Autodesk Inventor part; units mm, degrees
ref_plane "YZ Plane" through (0, 0, 0) normal (1, 0, 0) x (0, 1, 0)
ref_plane "XZ Plane" through (0, 0, 0) normal (0, 1, 0) x (-1, 0, 0)
ref_plane "XY Plane" through (0, 0, 0) normal (0, 0, 1) x (1, 0, 0)
ref_plane "Work Plane1" through (0, 0, 0) normal (0, 0, -1) x (-1, 0, 0)
sketch "Sketch16" plane through (0, 0, 0) normal (0, 0, -1) x (-1, 0, 0)
  line L0 (0, 0) -> (-76.2, 0)
  line L1 (-76.2, 0) -> (-101.6, 0)
  line L2 (-101.6, 0) -> (-101.6, 50.8)
  line L3 (-101.6, 50.8) -> (-76.2, 50.8)
  line L4 (-76.2, 50.8) -> (-76.2, 0)
  line L5 (-78.74, 48.26) -> (-99.06, 48.26)
  line L6 (-99.06, 48.26) -> (-99.06, 2.54)
  line L7 (-99.06, 2.54) -> (-78.74, 2.54)
  line L8 (-78.74, 2.54) -> (-78.74, 48.26)
  dimension "d54" = 25.4
  dimension "d55" = 50.8
  dimension "d56" = 2.54
  dimension "d57" = 2.54
  dimension "d58" = 2.54
  dimension "d59" = 2.54
extrude "Extrusion13" add sketch "Sketch16" against normal blind 152.4
ref_plane "Work Plane4" through (0, 0, 0) normal (0, 0, -1) x (-1, 0, 0)
ref_plane "Work Plane3" through (0, 0, 0) normal (0, -1, 0) x (1, 0, 0)
sketch "Sketch20" plane through (0, 0, 0) normal (0, -1, 0) x (1, 0, 0)
  circle A0 centre (88.9, 12.7) radius 2.5797
  circle A1 centre (63.5, 12.7) radius 2.5797
  circle A2 centre (38.1, 12.7) radius 2.5797
  line L0 (0, 25.4) -> (76.2, 25.4)
  circle A3 centre (88.9, 38.1) radius 2.5797
  circle A4 centre (88.9, 63.5) radius 2.5797
  line L1 (76.2, 25.4) -> (76.2, 152.4)
  line L2 (101.6, 0) -> (101.6, 152.4)
  point P0 (0, 0)
  dimension "d71" = 12.7
  dimension "d72" = 12.7
  dimension "d73" = 12.7
  dimension "d74" = 5.1594
  dimension "d75" = 5.1594
  dimension "d76" = 5.1594
  dimension "d77" = 12.7
  dimension "d78" = 12.7
  dimension "d79" = 5.1594
  dimension "d80" = 5.1594
  dimension "d81" = 12.7
  dimension "d82" = 25.4
  dimension "d83" = 25.4
  dimension "d84" = 25.4
  dimension "d85" = 25.4
extrude "Extrusion16" cut sketch "Sketch20" against normal blind 76.2
ref_plane "Work Plane2" through (0, 50.8, 25.4) normal (0, 1, 0) x (1, 0, 0)
sketch "Sketch24" plane through (0, 50.8, 25.4) normal (0, 1, 0) x (1, 0, 0)
  circle A0 centre (88.9, -114.3) radius 2.5797
  circle A1 centre (88.9, -88.9) radius 2.5797
  line L0 (101.6, -127) -> (76.2, -127)
  line L1 (76.2, 0) -> (76.2, -127)
  point P0 (0, 25.4)
  dimension "d112" = 12.7
  dimension "d113" = 25.4
  dimension "d114" = 5.1594
  dimension "d115" = 5.1594
  dimension "d116" = 12.7
  dimension "d117" = 12.7
extrude "Extrusion20" cut sketch "Sketch24" against normal blind 50.8
sketch "Sketch25" plane through (101.6, 0, 0) normal (1, 0, 0) x (0, 0, -1)
  point P0 (0, 0)
equation "\"d56\" = d48"
equation "\"d57\" = d48"
equation "\"d58\" = d48"
equation "\"d59\" = d48"
equation "\"d72\" = d71"
equation "\"d73\" = d71"
equation "\"d75\" = d74"
equation "\"d76\" = d74"
equation "\"d77\" = d71"
equation "\"d78\" = d71"
equation "\"d79\" = d74"
equation "\"d80\" = d74"
equation "\"d81\" = d71"
equation "\"d83\" = d82"
equation "\"d84\" = d82"
equation "\"d85\" = d82"
equation "\"d115\" = d114"
properties part number "right arm"
Source: CAD feature listing. Evaluate the final solid. Frame: model axes, mm. A direction names the side the tool comes from. Round coordinates to 2 decimals unless told otherwise and drop trailing zeros. Loops run counter-clockwise (first coordinate to the right, second up) from the corner with the lowest first, then second, coordinate; pieces in that order, holes last. Notation, with made-up numbers: (39, 84.5) - (63, 84.5) arc R22 ccw to (63, 106.5) - close; hole circle Ø5 at (34, 36.5). An arc over 180 degrees is marked (long way). Write item = value, one per line. Start each with the question number.
Item 1: Section query C-C on z = 139.7. Output: boundary loops of the cut face in (x, y).
Item 2: Material intervals for line 1 (Z direction, x = 88.9, y = 49.2); line 2 (X direction, y = 19.5, z = 93); line 3 (Y direction, x = 82.25, z = 89), sorted ascending.
Item 3: Mould query, pull axis X, two halves, no side actions, for faces 3 (the face through (101.6, 25, 75)), 4 (the face through (99.3, 27.4, 152.4)), 5 (the face through (89, 48.26, 75)). Classes: released by +X, released by -X, zero draft, split by the parting line, or undercut.
Item 4: Section query D-D on z = 119.5. Output: boundary loops of the cut face in (x, y).
Item 5: Section query B-B on x = 96.5. Output: boundary loops of the cut face in (y, z).
Item 6: Section query A-A on y = 43. Output: boundary loops of the cut face in (x, z).
Item 7: Reachability of faces 1 (the face through (99.06, 26, 75)), 2 (the face through (88.564, 1.252, 66.058)) from +Z, -Z, +X, -X, +Y, -Y: full face, straight path, thin tool, end or side. Return the list, or none.
Results list:
q1.outline = (76.2, 0) - (86.32, 0) - (86.32, 2.54) - (78.74, 2.54) - (78.74, 48.26) - (86.32, 48.26) - (86.32, 50.8) - (76.2, 50.8) - close; (91.48, 0) - (101.6, 0) - (101.6, 50.8) - (91.48, 50.8) - (91.48, 48.26) - (99.06, 48.26) - (99.06, 2.54) - (91.48, 2.54) - close
q2.line_1 = 0 to 10.12, 15.28 to 35.52, 40.68 to 60.92, 66.08 to 111.72, 116.88 to 137.12, 142.28 to 152.4
q2.line_2 = 76.2 to 78.74, 99.06 to 101.6
q2.line_3 = 0 to 2.54, 48.26 to 50.8
q3.face_3 = released by +X
q3.face_4 = zero draft
q3.face_5 = undercut
q4.outline = (76.2, 0) - (101.6, 0) - (101.6, 50.8) - (76.2, 50.8) - close; hole (78.74, 2.54) - (99.06, 2.54) - (99.06, 48.26) - (78.74, 48.26) - close
q5.outline = (0, 0) - (2.54, 0) - (2.54, 152.4) - (0, 152.4) - close; (48.26, 0) - (50.8, 0) - (50.8, 152.4) - (48.26, 152.4) - close
q6.outline = (76.2, 0) - (78.74, 0) - (78.74, 152.4) - (76.2, 152.4) - close; (99.06, 0) - (101.6, 0) - (101.6, 152.4) - (99.06, 152.4) - close
q7.face_1 = +Z, -Z
q7.face_2 = +Y, -Y
